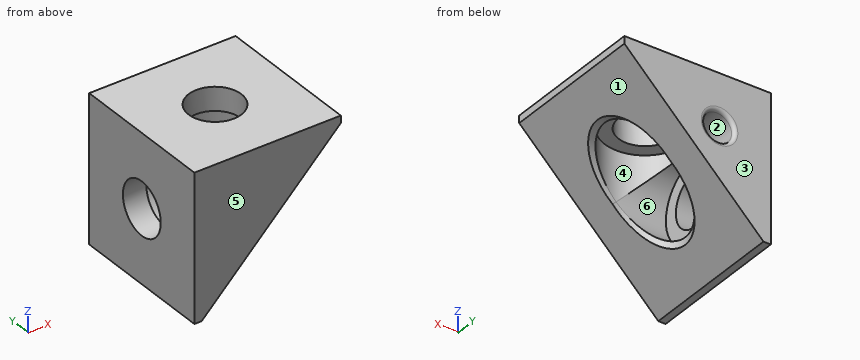
from build123d import *

# Parameters (mm, degrees)
BOSS_EXTRUDE1_DEPTH     = 10
CUT_EXTRUDE1_REACH      = 32
SKETCH3_R               = 3.6
CUT_EXTRUDE3_REACH      = 35.2
CUT_EXTRUDE3_START      = -3.2
SKETCH3_4_R             = 5.5
SKETCH3_4_R_2           = 3.6
CUT_EXTRUDE2_REACH      = 32
CUT_EXTRUDE2_END_RADIUS = 5.5
SKETCH4_R               = 3.6
CUT_EXTRUDE4_REACH      = 35.2
CUT_EXTRUDE4_START      = -3.2
SKETCH4_3_R             = 5.5
SKETCH4_3_R_2           = 3.6
SKETCH5_R               = 2
CUT_EXTRUDE5_DEPTH      = 4.5
FILLET1_R               = 0.5


with BuildPart() as part:
    # Sketch2 → Boss-Extrude1 (new, symmetric)
    with BuildSketch(Plane(origin=(0, 0, 0), x_dir=(1, 0, 0), z_dir=(0, 1, 0))):
        Polygon((0, 0), (0, 20), (1, 20), (20, 1), (20, 0), align=None)
    extrude(amount=BOSS_EXTRUDE1_DEPTH, both=True)

    # Cut-Extrude1: up to this plane
    cut_extrude1_end = Plane(origin=(1, 10, -20), z_dir=(-0.7071067811865476, 0, 0.7071067811865476))
    # Sketch3 → Cut-Extrude1 (cut, up to the surface)
    with BuildSketch(Plane.XY, mode=Mode.PRIVATE) as cut_extrude1_sk1:
        with Locations((10, 0)):
            Circle(SKETCH3_R)
    cut_extrude1_tool1 = split(extrude(cut_extrude1_sk1.sketch, amount=-CUT_EXTRUDE1_REACH, mode=Mode.PRIVATE), bisect_by=cut_extrude1_end, keep=Keep.BOTH, mode=Mode.PRIVATE)
    add(cut_extrude1_tool1.solids().sort_by_distance((10, 0, 0))[0], mode=Mode.SUBTRACT)

    # Cut-Extrude3: up to this plane
    cut_extrude3_end = Plane(origin=(1, 10, -20), z_dir=(-0.7071067811865476, 0, 0.7071067811865476))
    # Sketch3_4 → Cut-Extrude3 (cut, up to the surface)
    with BuildSketch(Plane.XY.offset(CUT_EXTRUDE3_START), mode=Mode.PRIVATE) as cut_extrude3_sk1:
        with Locations((10, 0)):
            Circle(SKETCH3_4_R)
        with Locations((10, 0)):
            Circle(SKETCH3_4_R_2, mode=Mode.SUBTRACT)
    cut_extrude3_tool1 = split(extrude(cut_extrude3_sk1.sketch, amount=-CUT_EXTRUDE3_REACH, mode=Mode.PRIVATE), bisect_by=cut_extrude3_end, keep=Keep.BOTH, mode=Mode.PRIVATE)
    add(cut_extrude3_tool1.solids().sort_by_distance((4.655563, 0, -3.2))[0], mode=Mode.SUBTRACT)

    # Cut-Extrude2: up to this cylinder (the profile starts outside it)
    cut_extrude2_end = Plane(origin=(10, 0, -10), z_dir=(0, 0, 1)) * Cylinder(CUT_EXTRUDE2_END_RADIUS, 76, mode=Mode.PRIVATE)
    # Sketch4 → Cut-Extrude2 (cut, up to the surface)
    with BuildSketch(Plane.ZY, mode=Mode.PRIVATE) as cut_extrude2_sk1:
        with Locations((-10, 0)):
            Circle(SKETCH4_R)
    cut_extrude2_tool1 = extrude(cut_extrude2_sk1.sketch, amount=-CUT_EXTRUDE2_REACH, mode=Mode.PRIVATE) - cut_extrude2_end
    add(cut_extrude2_tool1.solids().sort_by_distance((0, 0, -10))[0], mode=Mode.SUBTRACT)

    # Cut-Extrude4: up to this plane
    cut_extrude4_end = Plane(origin=(1, 10, -20), z_dir=(-0.7071067811865476, 0, 0.7071067811865476))
    # Sketch4_3 → Cut-Extrude4 (cut, up to the surface)
    with BuildSketch(Plane.ZY.offset(CUT_EXTRUDE4_START), mode=Mode.PRIVATE) as cut_extrude4_sk1:
        with Locations((-10, 0)):
            Circle(SKETCH4_3_R)
        with Locations((-10, 0)):
            Circle(SKETCH4_3_R_2, mode=Mode.SUBTRACT)
    cut_extrude4_tool1 = split(extrude(cut_extrude4_sk1.sketch, amount=-CUT_EXTRUDE4_REACH, mode=Mode.PRIVATE), bisect_by=cut_extrude4_end, keep=Keep.BOTH, mode=Mode.PRIVATE)
    add(cut_extrude4_tool1.solids().sort_by_distance((3.2, 0, -15.344437))[0], mode=Mode.SUBTRACT)

    # Sketch5 → Cut-Extrude5 (cut)
    with BuildSketch(Plane(origin=(0, 10, 0), x_dir=(1, 0, 0), z_dir=(0, 1, 0))):
        with Locations(Location((7, 7, 0), (0, 0, 270))):
            Circle(SKETCH5_R)
    extrude(amount=-CUT_EXTRUDE5_DEPTH, mode=Mode.SUBTRACT)

    # Fillet1
    fillet1_edges = [part.edges().sort_by_distance(p)[0] for p in [
        (7, 10, -9),
    ]]
    fillet(fillet1_edges, radius=FILLET1_R)


solid = part.part
Here's how the part is built. I have some questions about the finished solid (model axes, mm). Face numbers are marked on the shaded views. A direction names the side the tool comes from. Coordinates: 2 decimals unless noted, no trailing zeros. Order: outer loops, then holes, each group sorted by start corner. A loop starts at its lowest first (then second) coordinate and runs counter-clockwise, first axis right, second up.
Item 1: If we section it at B-B on x = 12.25: List the corners of the cut face in (y, z) for me, plus the area to 3 significant figures.
Result sheet:
outline: (-10, -8.75) - (-5.36, -8.75) arc R5.5 cw to (-5.02, -7.75) - (-5.02, -3.2) - (-2.81, -3.2) - (-2.81, 0) - (-10, 0) - close; (2.81, -3.2) - (5.02, -3.2) - (5.02, -7.75) arc R5.5 cw to (5.36, -8.75) - (10, -8.75) - (10, 0) - (2.81, 0) - close
area: 101 mm2
Item 2: If we section it at C-C on y = 2: List the corners of the cut face in (x, z) for me.
Result sheet:
outline: (0, -20) - (1, -20) - (4.88, -16.12) - (4.88, -15.12) - (3.2, -15.12) - (3.2, -12.99) - (0, -12.99) - close; (0, -7.01) - (3.2, -7.01) - (3.2, -4.88) - (4.88, -4.88) - (4.88, -3.2) - (7.01, -3.2) - (7.01, 0) - (0, 0) - close; (12.99, -3.2) - (15.12, -3.2) - (15.12, -4.88) - (16.12, -4.88) - (20, -1) - (20, 0) - (12.99, 0) - close
Item 3: If we section it at A-A on z = -7: List the corners of the cut face in (x, y) for me, plus the area to 3 significant figures.
Result sheet:
outline: (0, -10) - (14, -10) - (14, -4.61) - (13, -4.61) arc R5.5 cw to (7, -4.61) - (3.2, -4.61) - (3.2, -1.99) - (0, -1.99) - close; (0, 1.99) - (3.2, 1.99) - (3.2, 4.61) - (7, 4.61) arc R5.5 cw to (13, 4.61) - (14, 4.61) - (14, 10) - (9.5, 10) arc R0.5 ccw to (9, 9.5) - (9, 5.5) - (5, 5.5) - (5, 9.5) arc R0.5 ccw to (4.5, 10) - (0, 10) - close
area: 142 mm2
Item 4: I need wall thicknesses on line 1 (Y direction, x = 6.5, z = -10); line 2 (Z direction, x = 6.5, y = 1.25); line 3 (Y direction, x = 1.5, z = -12.25). Which ranges of each line are inside material? Lowest first, please.
Result sheet:
line 1: y = -10 to -5.5, 5.5 to 10
line 2: z = -3.2 to 0
line 3: y = -10 to -2.81, 2.81 to 10
Item 5: For the marked faces 4, 5 and 6, which set-ups out of +Z, -Z, +X, -X, +Y, -Y let a thin tool reach every point of the face, with its end or its side?
Result sheet:
face 4: -Z
face 5: +Z, -Z, +X, -X, -Y
face 6: +X
Item 6: For P1, Ø3.5, axis at y = 1.5, z = -12.5, coming from the +X side; P2, Ø12, axis at x = 8, y = -1, coming from the -Z side; P3, Ø3, axis at x = 15, y = -6.5, coming from the -Z side, each with a flat end and sliding along its axis, tell me the tip position at first contact or that it passes through.
Result sheet:
P1: stops at x = 3.2
P2: stops at z = -19
P3: stops at z = -7.5
Item 7: If we mould it in two halves opening along Z, with no side actions, what happens to the marked faces 1, 2 and 3? For each: +Z half, -Z half, draft (parallel to the pull), parting line (faces both ways), or undercut.
Result sheet:
face 1: -Z half
face 2: undercut
face 3: draft
Item 8: If we section it at D-D on z = -3.75: List the corners of the cut face in (x, y) for me.
Result sheet:
outline: (0, -10) - (17.25, -10) - (17.25, 10) - (0, 10) - close; hole circle Ø11 at (10, 0)
